The drawing under review shows one solid part. Ordinate dimensions are in mm from its lowest x, y, z. Coordinates: 2 decimals unless noted, no trailing zeros. Order: outer loops, then holes, each group sorted by start corner. A loop starts at its lowest first (then second) coordinate and runs counter-clockwise, first axis right, second up. Notation, with made-up numbers: (-3.5, -15) -> (14.5, -15) arc R18 cw to (14.5, 3) -> close; hole circle Ø10 at (13.25, 87). An arc over 180 degrees is marked (long way). Use one line per item in the form item = value.
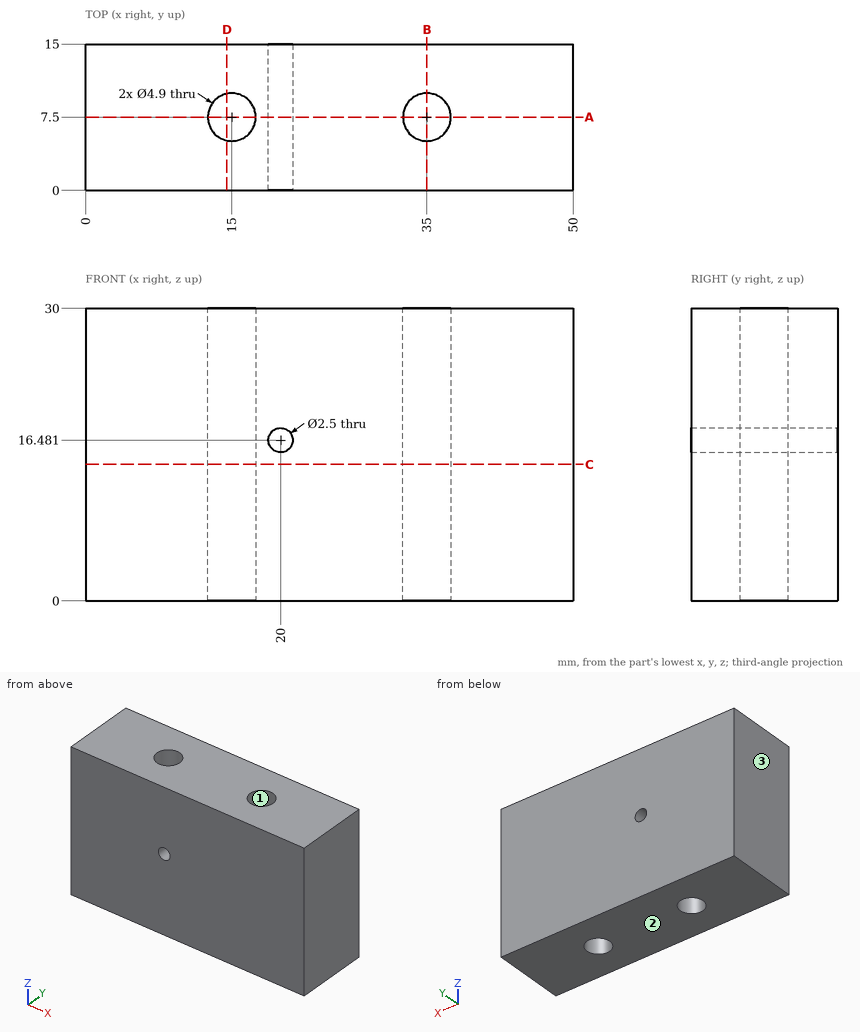
Item 1: We need section D-D (x = 14.5). Write out the cut boundary in (y, z), plus the area to 3 significant figures.
Results found:
outline = (0, 0) -> (5.1, 0) -> (5.1, 30) -> (0, 30) -> close; (9.9, 0) -> (15, 0) -> (15, 30) -> (9.9, 30) -> close
area = 306 mm²
Item 2: Draft analysis for pull direction X (two halves, no side actions). For the marked faces 1, 2 and 3, state which applies: released by +X, released by -X, zero draft, split by the parting line, or undercut.
Results found:
face_1 = undercut
face_2 = zero draft
face_3 = released by -X
Item 3: We need section B-B (x = 35). Write out the cut boundary in (y, z).
Results found:
outline = (0, 0) -> (5.05, 0) -> (5.05, 30) -> (0, 30) -> close; (9.95, 0) -> (15, 0) -> (15, 30) -> (9.95, 30) -> close
Item 4: We need section C-C (z = 14). Write out the cut boundary in (x, y).
Results found:
outline = (0, 0) -> (50, 0) -> (50, 15) -> (0, 15) -> close; hole circle Ø4.9 at (15, 7.5); hole circle Ø4.9 at (35, 7.5)
Item 5: To check wall thickness, follow L1, parallel to Y at x = 35, z = 21; L2, parallel to X at y = 9, z = 3.75; L3, parallel to X at y = 7, z = 2.75. State the ranges of each line that lie inside material, in increasing order. Write a range as from..to.
Results found:
L1 = 0..5.05, 9.95..15
L2 = 0..13.06, 16.94..33.06, 36.94..50
L3 = 0..12.6, 17.4..32.6, 37.4..50
Item 6: We need section A-A (y = 7.5). Write out the cut boundary in (x, z).
Results found:
outline = (0, 0) -> (12.55, 0) -> (12.55, 30) -> (0, 30) -> close; (17.45, 0) -> (32.55, 0) -> (32.55, 30) -> (17.45, 30) -> close; (37.45, 0) -> (50, 0) -> (50, 30) -> (37.45, 30) -> close; hole circle Ø2.5 at (20, 16.48)
Item 7: Clearance check with a flat-ended pin moving along its axis: pin 1 (4.5 mm diameter, centred on x = 15, y = 7.5, fed in from -Z). State where the tip first meets the part, or that it passes through.
Results found:
pin_1 = through
